Here's how the part is built. I have some questions about the finished solid (model axes, mm). Face numbers are marked on the shaded views. A direction names the side the tool comes from. Round coordinates to 2 decimals unless told otherwise and drop trailing zeros. Order: outer loops, then holes, each group sorted by start corner. A loop starts at its lowest first (then second) coordinate and runs counter-clockwise, first axis right, second up. Notation, with made-up numbers: (19.5, 21) -> (68.5, 21) arc R31 cw to (68.5, 46) -> close; hole circle Ø8 at (62.5, 61). An arc over 180 degrees is marked (long way). Answer in a Markdown table with one row per item.
```python
from build123d import *

# Parameters (mm, degrees)
F1_DEPTH = 8.128
F2_R     = 5.08
F3_R     = 0.508


with BuildPart() as f1:
    # F0 (on Top) → F1 (new body)
    with BuildSketch(Plane.XY):
        with BuildLine():
            ThreePointArc((9.7169721006, 19.05), (-13.6068060839, 9.525), (9.7169721006, 0))
            Line((9.7169721006, 0), (38.1, 0))
            Line((38.1, 0), (38.1, 19.05))
            Line((38.1, 19.05), (9.7169721006, 19.05))
        make_face()
    extrude(amount=F1_DEPTH)

    # F2
    f2_edges = [f1.edges().sort_by_distance(p)[0] for p in [
        (38.1, 19.05, 4.064),
        (38.1, 0, 4.064),
    ]]
    fillet(f2_edges, radius=F2_R)

    # F3
    f3_edges = [f1.edges().sort_by_distance(p)[0] for p in [
        (-13.606806, 9.525, 8.128),
        (21.368486, 0, 8.128),
        (36.612102, 1.487898, 8.128),
        (38.1, 9.525, 8.128),
        (36.612102, 17.562102, 8.128),
        (21.368486, 19.05, 8.128),
        (-13.606806, 9.525, 0),
        (21.368486, 0, 0),
        (36.612102, 1.487898, 0),
        (38.1, 9.525, 0),
        (21.368486, 19.05, 0),
        (36.612102, 17.562102, 0),
    ]]
    fillet(f3_edges, radius=F3_R)


solid = f1.part
```
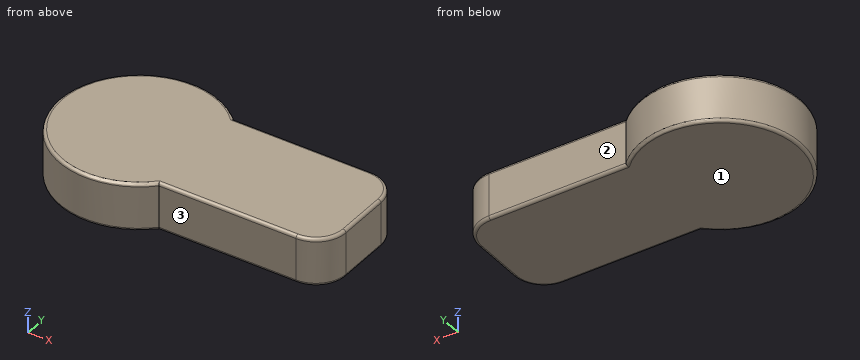
1. For the marked faces 1, 2 and 3, which set-ups out of +Z, -Z, +X, -X, +Y, -Y let a thin tool reach every point of the face, with its end or its side?
Numbers:
| item | result |
|---|---|
| face 1 | -Z, +X, -X, +Y, -Y |
| face 2 | +Z, -Z, +X, +Y |
| face 3 | +Z, -Z, +X, -Y |
2. Suppose I cut it at B-B on x = 23.5. Write out the boundary of the cut face in (y, z), then the cut area to 3 significant figures.
Numbers:
| item | result |
|---|---|
| outline | (0, 0.51) arc R0.51 ccw to (0.51, 0) -> (18.54, 0) arc R0.51 ccw to (19.05, 0.51) -> (19.05, 7.62) arc R0.51 ccw to (18.54, 8.13) -> (0.51, 8.13) arc R0.51 ccw to (0, 7.62) -> close |
| area | 155 mm2 |
3. For pin 1 Ø2 at (y, z) = (4.5, 4) entering from -X; pin 2 Ø2 at (x, z) = (-7.5, 1.5) entering from +Y; pin 3 Ø3.5 at (x, z) = (16.5, 4.5) entering from -Y, each with a flat end and sliding along its axis, tell me the tip position at first contact or that it passes through.
Numbers:
| item | result |
|---|---|
| pin 1 | stops at x = -13 |
| pin 2 | stops at y = 21.48 |
| pin 3 | stops at y = 0 |
4. Suppose I cut it at A-A on z = 2.5. Write out the boundary of the cut face in (x, y) (3 decimals), then the cut area to 3 significant figures.
Numbers:
| item | result |
|---|---|
| outline | (9.717, 0) -> (33.02, 0) arc R5.08 ccw to (38.1, 5.08) -> (38.1, 13.97) arc R5.08 ccw to (33.02, 19.05) -> (9.717, 19.05) arc R13.607 ccw (long way) to start |
| area | 1,060 mm2 |
5. Please list where these lines run through material, in increasing order: line 1 along Y through (x, z) = (27.5, 5.5); line 2 along X through (y, z) = (9.75, 3).
Numbers:
| item | result |
|---|---|
| line 1 | y = 0 to 19.05 |
| line 2 | x = -13.6 to 38.1 |
